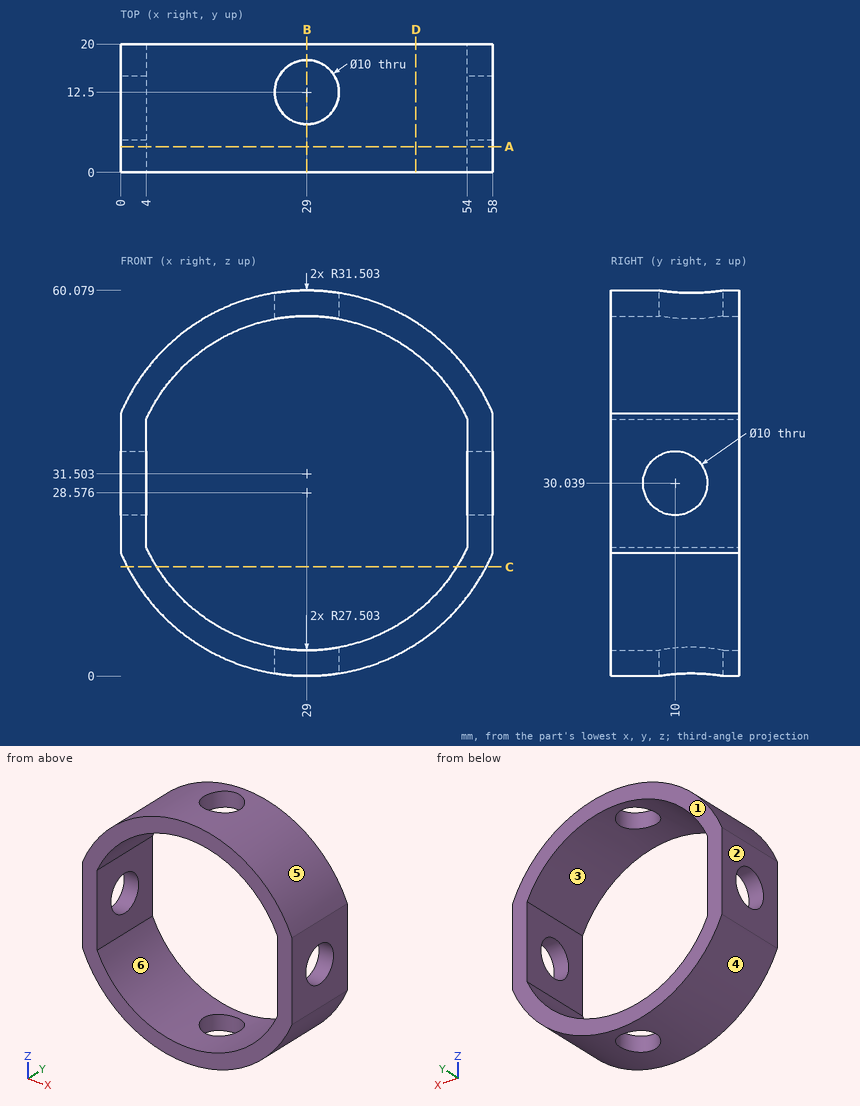
Can you work these out from the drawing? Everything is in mm from the part's minimum corner. A direction names the side the tool comes from. Give positions to 0.01 mm unless a question says otherwise; leave off trailing zeros. Order: outer loops, then holes, each group sorted by start corner. A loop starts at its lowest first (then second) coordinate and runs counter-clockwise, first axis right, second up. Notation, with made-up numbers: M 61.25,56.25 L 99.25,56.25 A13 cw 99.25,71.25 Z; hole C 8.25,83 d10. An arc over 180 degrees is marked long. Use a Markdown table: item, result. Add a question column.
Item 1: Suppose I cut it at B-B (x = 29). List the corners of the cut face in (y, z) for me.
Item 2: For the marked faces 5 and 6, which set-ups out of +Z, -Z, +X, -X, +Y, -Y let a thin tool reach every point of the face, with its end or its side?
Item 3: We'd pull the mould along X, two halves only. Please class the marked faces 1, 2, 3 and 4: +X half, -X half, draft (parallel to the pull), parting line (faces both ways), or undercut.
Item 4: Suppose I cut it at D-D (x = 46). List the corners of the cut face in (y, z) for me (1 decimal).
Item 5: Will these pins go through, and if not, where does the flat tip stop? pin 1 (6 mm diameter, centred on x = 25, y = 7.5, fed in from +Z); pin 2 (8 mm diameter, centred on y = 10, z = 30.04, fed in from -X); pin 3 (2 mm diameter, centred on y = 3, z = 48.5, fed in from -X) (1 decimal); pin 4 (4 mm diameter, centred on y = 4.5, z = 47.5, fed in from +X).
Item 6: Suppose I cut it at C-C (z = 17). List the corners of the cut face in (x, y) for me, then the cut area to 3 significant figures.
Item 7: If I drill on L1, parallel to Y at x = 29, z = 58; L2, parallel to X at y = 17.75, z = 39; L3, parallel to X at y = 4, z = 44, over which ranges is the centre line in solid material (lowest first)? Write a range as [from, to].
Item 8: Suppose I cut it at A-A (y = 4). List the corners of the cut face in (x, z) for me (1 decimal).
Answer sheet:
| question | item | result |
|---|---|---|
| 1 | outline | M 0,0 L 7.5,0 L 7.5,4 L 0,4 Z; M 0,56.08 L 7.5,56.08 L 7.5,60.08 L 0,60.08 Z; M 17.5,0 L 20,0 L 20,4 L 17.5,4 Z; M 17.5,56.08 L 20,56.08 L 20,60.08 L 17.5,60.08 Z |
| 2 | face 5 | +Z, +Y, -Y |
| 2 | face 6 | +Y, -Y |
| 3 | face 1 | draft |
| 3 | face 2 | -X half |
| 3 | face 3 | undercut |
| 3 | face 4 | parting line |
| 4 | outline | M 0,5 L 20,5 L 20,9.9 L 0,9.9 Z; M 0,50.2 L 20,50.2 L 20,55.1 L 0,55.1 Z |
| 5 | pin 1 | stops at z = 60.06 |
| 5 | pin 2 | passes through |
| 5 | pin 3 | stops at x = 3.8 |
| 5 | pin 4 | stops at x = 55.57 |
| 6 | outline | M 1.03,0 L 5.63,0 L 5.63,20 L 1.03,20 Z; M 52.37,0 L 56.97,0 L 56.97,20 L 52.37,20 Z |
| 6 | area | 184 mm² |
| 7 | L1 | y = [0, 7.5], [17.5, 20] |
| 7 | L2 | x = [0, 4], [54, 58] |
| 7 | L3 | x = [1.53, 6.23], [51.77, 56.47] |
| 8 | outline | M 0,19.2 A31.5 ccw 58,19.2 L 58,40.9 A31.5 ccw 0,40.9 Z; hole M 4,20 A27.5 ccw 54,20 L 54,40 A27.5 ccw 4,40 Z |
